Could you check a few things on this model? Use its own coordinates, in mm. A direction names the side the tool comes from. Round coordinates to 2 decimals unless told otherwise and drop trailing zeros. Write each loop counter-clockwise with the first axis right and the second up, starting at its lowest first coordinate (ties: lowest second). Pieces come first, ordered by that corner, then holes. Notation, with made-up numbers: (42.25, -34) -> (97.25, -34) arc R32 ccw to (97.25, -1) -> close; hole circle Ø3 at (-1, 37). An arc over 180 degrees is marked (long way). Answer in a Markdown table with one row per item.
from build123d import *

# Parameters (mm, degrees)
SKETCH1_W                                       = 6.4
SKETCH1_H                                       = 172.8
BOSS_EXTRUDE1_DEPTH                             = 3.75
CHAMFER4_SIZE                                   = 5
CHAMFER4_SIZE2                                  = 3.501037691
FILLET1_R                                       = 0.5
SKETCH2_W                                       = 4.3
SKETCH2_H                                       = 152.8
BOSS_EXTRUDE2_DEPTH                             = 4.1
CSK_FOR_M2_FLAT_HEAD_MACHINE_SCREW1_D           = 2.4
CSK_FOR_M2_FLAT_HEAD_MACHINE_SCREW1_CSINK_D     = 4.4
CSK_FOR_M2_FLAT_HEAD_MACHINE_SCREW1_CSINK_ANGLE = 90
LPATTERN1_COUNT                                 = 3
LPATTERN1_PITCH                                 = 25
LPATTERN1_COL_COUNT                             = 3
LPATTERN1_COL_PITCH                             = 25


with BuildPart() as part:
    # Sketch1 → Boss-Extrude1 (new body)
    with BuildSketch(Plane(origin=(0, 0, 0), x_dir=(1, 0, 0), z_dir=(0, 1, 0))):
        with Locations((0, -76.4)):
            Rectangle(SKETCH1_W, SKETCH1_H)
    extrude(amount=BOSS_EXTRUDE1_DEPTH)

    # Chamfer4
    chamfer4_edges = [part.edges().sort_by_distance(p)[0] for p in [
        (0, 3.75, 162.8),
        (0, 3.75, -10),
    ]]
    chamfer4_side = [part.faces().sort_by_distance(p)[0] for p in [
        (0, 3.75, 76.4),
    ]]
    chamfer(chamfer4_edges, length=CHAMFER4_SIZE, length2=CHAMFER4_SIZE2, reference=chamfer4_side[0])

    # Fillet1
    fillet1_edges = [part.edges().sort_by_distance(p)[0] for p in [
        (-3.2, 3.75, 76.4),
        (3.2, 3.75, 76.4),
    ]]
    fillet(fillet1_edges, radius=FILLET1_R)

    # Sketch2 → Boss-Extrude2 (add)
    with BuildSketch(Plane(origin=(0, 3.75, 0), x_dir=(1, 0, 0), z_dir=(0, 1, 0))):
        with Locations((0, -76.4)):
            Rectangle(SKETCH2_W, SKETCH2_H)
    extrude(amount=BOSS_EXTRUDE2_DEPTH)

    # CSK for M2 Flat Head Machine Screw1 (through all)
    with Locations(Plane.XZ):
        with Locations((0, 76.4)):
            csk_for_m2_flat_head_machine_screw1 = CounterSinkHole(CSK_FOR_M2_FLAT_HEAD_MACHINE_SCREW1_D / 2, CSK_FOR_M2_FLAT_HEAD_MACHINE_SCREW1_CSINK_D / 2, counter_sink_angle=CSK_FOR_M2_FLAT_HEAD_MACHINE_SCREW1_CSINK_ANGLE)

    # LPattern1: CSK for M2 Flat Head Machine Screw1 ×3
    with Locations(*[(0, 0, -i * LPATTERN1_PITCH) for i in range(1, LPATTERN1_COUNT)]):
        add(csk_for_m2_flat_head_machine_screw1, mode=Mode.SUBTRACT)

    # LPattern1 col: CSK for M2 Flat Head Machine Screw1 ×3
    with Locations(*[(0, 0, i * LPATTERN1_COL_PITCH) for i in range(1, LPATTERN1_COL_COUNT)]):
        add(csk_for_m2_flat_head_machine_screw1, mode=Mode.SUBTRACT)


solid = part.part
1) Imagine slicing it at A-A, the plane y = 5.75. Please give me the cut outline in (x, z).
Findings:
| item | result |
|---|---|
| outline | (-2.15, 0) -> (2.15, 0) -> (2.15, 152.8) -> (-2.15, 152.8) -> close; hole circle Ø2.4 at (0, 26.4); hole circle Ø2.4 at (0, 51.4); hole circle Ø2.4 at (0, 76.4); hole circle Ø2.4 at (0, 101.4); hole circle Ø2.4 at (0, 126.4) |
2) Imagine slicing it at C-C, the plane x = 0. Count the separate pieces of the cut face and the enclosed holes in it, plus the area to 3 significant figures.
Findings:
| item | result |
|---|---|
| separate pieces | 6 |
| enclosed holes | 0 |
| area | 1,160 mm^2 |
3) For faces 1 (the face through (0, 6, 152.8)), 2 (the face through (2.15, 6, 77)), 3 (the face through (0, 6, 0)), 4 (the face through (-2.15, 6, 77)), which set-ups out of +Z, -Z, +X, -X, +Y, -Y let a thin tool reach every point of the face, with its end or its side?
Findings:
| item | result |
|---|---|
| face 1 | +Z, +X, -X, +Y |
| face 2 | +Z, -Z, +X, +Y |
| face 3 | -Z, +X, -X, +Y |
| face 4 | +Z, -Z, -X, +Y |
4) Please list where these lines run through material, in increasing order: line 1 (Z direction, x = 0, y = 5); line 2 (X direction, y = 4.25, z = 101.4); line 3 (Z direction, x = -1, y = 6).
Findings:
| item | result |
|---|---|
| line 1 | z = 0 to 25.2, 27.6 to 50.2, 52.6 to 75.2, 77.6 to 100.2, 102.6 to 125.2, 127.6 to 152.8 |
| line 2 | x = -2.15 to -1.2, 1.2 to 2.15 |
| line 3 | z = 0 to 25.74, 27.06 to 50.74, 52.06 to 75.74, 77.06 to 100.74, 102.06 to 125.74, 127.06 to 152.8 |
5) Imagine slicing it at B-B, the plane z = 96. Please give me the cut outline in (x, y), plus the area to 3 significant figures.
Findings:
| item | result |
|---|---|
| outline | (-3.2, 0) -> (3.2, 0) -> (3.2, 3.25) arc R0.5 ccw to (2.7, 3.75) -> (2.15, 3.75) -> (2.15, 7.85) -> (-2.15, 7.85) -> (-2.15, 3.75) -> (-2.7, 3.75) arc R0.5 ccw to (-3.2, 3.25) -> close |
| area | 41.5 mm^2 |
6) For pin 1 (1.5 mm diameter, centred on x = -0.5, y = 2, fed in from -Z); pin 2 (2 mm diameter, centred on y = 5.5, z = 106.5, fed in from +X); pin 3 (3 mm diameter, centred on x = 0, z = 26.4, fed in from -Y), each with a flat end and sliding along its axis, tell me the tip position at first contact or that it passes through.
Findings:
| item | result |
|---|---|
| pin 1 | stops at z = -8.57 |
| pin 2 | stops at x = 2.15 |
| pin 3 | stops at y = 0.7 |
